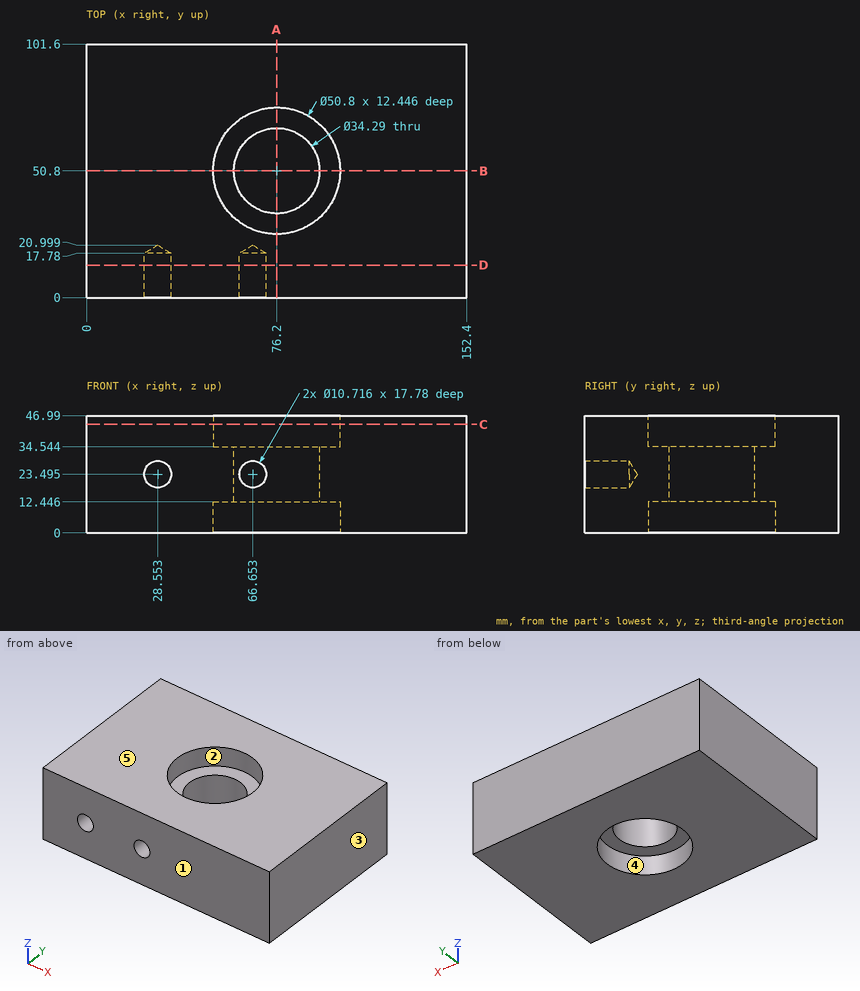
Job drawing, mm, ordinate dimensions from the low corner. One solid piece. A direction names the side the tool comes from. Round coordinates to 2 decimals unless told otherwise and drop trailing zeros. Write each loop counter-clockwise with the first axis right and the second up, starting at its lowest first coordinate (ties: lowest second). Pieces come first, ordered by that corner, then holes.
1) Band-saw the part on A-A, the plane x = 76.2. List the corners of the cut face in (y, z) (1 decimal).
2) Band-saw the part on B-B, the plane y = 50.8. List the corners of the cut face in (x, z) (1 decimal).
3) Band-saw the part on D-D, the plane y = 13. List the corners of the cut face in (x, z) (1 decimal).
4) Mould opens along X. For the marked faces 3, 4 and 5 say: +X half, -X half, draft (parallel to the pull), parting line (faces both ways), or undercut.
5) 3-axis set-ups, long thin cutter, end or side, ignore diameter. For the marked faces 1 and 2: which of +Z, -Z, +X, -X, +Y, -Y reach the whole face in a straight line?
6) Pin check, flat tips, straight feed: pin 1 (10 mm diameter, centred on x = 76, z = 10.5, fed in from -Y); pin 2 (9.5 mm diameter, centred on x = 66.65, z = 23.5, fed in from -Y); pin 3 (15 mm diameter, centred on x = 75.5, y = 38.5, fed in from +Z). Stop position of each tip, or through.
7) Drill centre lines: probe 1 along X at (y, z) = (51.5, 43); probe 2 along Y at (x, z) = (76, 24); probe 3 along Y at (x, z) = (55.5, 39). Where is each one in solid material? Low to high.
8) Band-saw the part on C-C, the plane z = 43.5. List the corners of the cut face in (x, y).
Ans:
1. outline: (0, 0) - (25.4, 0) - (25.4, 12.4) - (33.7, 12.4) - (33.7, 34.5) - (25.4, 34.5) - (25.4, 47) - (0, 47) - close; (67.9, 12.4) - (76.2, 12.4) - (76.2, 0) - (101.6, 0) - (101.6, 47) - (76.2, 47) - (76.2, 34.5) - (67.9, 34.5) - close
2. outline: (0, 0) - (50.8, 0) - (50.8, 12.4) - (59.1, 12.4) - (59.1, 34.5) - (50.8, 34.5) - (50.8, 47) - (0, 47) - close; (93.3, 12.4) - (101.6, 12.4) - (101.6, 0) - (152.4, 0) - (152.4, 47) - (101.6, 47) - (101.6, 34.5) - (93.3, 34.5) - close
3. outline: (0, 0) - (152.4, 0) - (152.4, 47) - (0, 47) - close; hole circle Ø10.7 at (28.6, 23.5); hole circle Ø10.7 at (66.7, 23.5)
4. face 3: +X half
4. face 4: undercut
4. face 5: draft
5. face 1: +Z, -Z, +X, -X, -Y
5. face 2: +Z
6. pin 1: stops at y = 0
6. pin 2: stops at y = 18.14
6. pin 3: stops at z = 34.54
7. probe 1: x = 0 to 50.81, 101.59 to 152.4
7. probe 2: y = 0 to 33.66, 67.94 to 101.6
7. probe 3: y = 0 to 36.08, 65.52 to 101.6
8. outline: (0, 0) - (152.4, 0) - (152.4, 101.6) - (0, 101.6) - close; hole circle Ø50.8 at (76.2, 50.8)
